```python
from build123d import *

# Parameters (mm, degrees)
SKETCH1_W                                        = 101.6
SKETCH1_H                                        = 50.8
BOSS_EXTRUDE1_DEPTH                              = 25.4
SKETCH2_R                                        = 22.225
CUT_EXTRUDE1_DEPTH                               = 6.35
SKETCH3_R                                        = 9.525
CUT_EXTRUDE2_DEPTH                               = 7.9375
F_1_2_20_TAPPED_HOLE1_D                          = 11.50874
CBORE_FOR_1_2_SOCKET_HEAD_CAP_SCREW1_D           = 13.49248
CBORE_FOR_1_2_SOCKET_HEAD_CAP_SCREW1_CBORE_D     = 20.6375
CBORE_FOR_1_2_SOCKET_HEAD_CAP_SCREW1_CBORE_DEPTH = 12.7


with BuildPart() as part:
    # Sketch1 → Boss-Extrude1 (new body)
    with BuildSketch(Plane(origin=(0, 0, 0), x_dir=(0, 0, -1), z_dir=(1, 0, 0))):
        with Locations((50.8, 25.4)):
            Rectangle(SKETCH1_W, SKETCH1_H)
    extrude(amount=BOSS_EXTRUDE1_DEPTH)

    # Sketch2 → Cut-Extrude1 (cut)
    with BuildSketch(Plane(origin=(0, 50.8, 0), x_dir=(1, 0, 0), z_dir=(0, 1, 0))):
        with Locations((12.7, 50.8)):
            Circle(SKETCH2_R)
    extrude(amount=-CUT_EXTRUDE1_DEPTH, mode=Mode.SUBTRACT)

    # Sketch3 → Cut-Extrude2 (cut)
    with BuildSketch(Plane(origin=(0, 44.45, 0), x_dir=(1, 0, 0), z_dir=(0, 1, 0))):
        with Locations(Location((12.7, 50.8, 0), (0, 0, 270))):
            Circle(SKETCH3_R)
    extrude(amount=-CUT_EXTRUDE2_DEPTH, mode=Mode.SUBTRACT)

    # 1/2-20 Tapped Hole1 (through all)
    with Locations(Plane(origin=(0, 36.5125, 0), x_dir=(1, 0, 0), z_dir=(0, 1, 0))):
        with Locations((12.7, 50.8)):
            Hole(F_1_2_20_TAPPED_HOLE1_D / 2)

    # CBORE for 1/2 Socket Head Cap Screw1 (through all)
    with Locations(Plane(origin=(0, 50.8, 0), x_dir=(1, 0, 0), z_dir=(0, 1, 0))):
        with Locations((12.7, 88.9), (12.7, 12.7)):
            CounterBoreHole(CBORE_FOR_1_2_SOCKET_HEAD_CAP_SCREW1_D / 2, CBORE_FOR_1_2_SOCKET_HEAD_CAP_SCREW1_CBORE_D / 2, CBORE_FOR_1_2_SOCKET_HEAD_CAP_SCREW1_CBORE_DEPTH)


solid = part.part
```
Could you check a few things on this model? Use its own coordinates, in mm. A direction names the side the tool comes from. Coordinates: 2 decimals unless noted, no trailing zeros. Order: outer loops, then holes, each group sorted by start corner. A loop starts at its lowest first (then second) coordinate and runs counter-clockwise, first axis right, second up. Notation, with made-up numbers: M -6,76.25 L 36,76.25 A20 cw 36,92.25 Z; hole C -12,44.25 d4. An arc over 180 degrees is marked long. Use one line per item in the form item = value. Start each with the question number.
1. Suppose I cut it at B-B on z = -88.9. Write out the boundary of the cut face in (x, y).
2. Please list where these lines run through material, in increasing order: line 1 (Z direction, x = 12.7, y = 44.5) (3 decimals); line 2 (Z direction, x = 15.5, y = 6); line 3 (X direction, y = 14.5, z = -88.9).
3. For pin 1 (4 mm diameter, centred on x = 10, z = -47.5, fed in from +Y); pin 2 (4 mm diameter, centred on x = 23, z = -90, fed in from -Y); pin 3 (10.5 mm diameter, centred on x = 12, z = -84.5, fed in from +Y), each with a flat end and sliding along its axis, tell me the tip position at first contact or that it passes through.
4. Suppose I cut it at D-D on y = 16. Write out the boundary of the cut face in (x, z), then the cut area to 3 significant figures.
5. On a 3-axis mill with a long thin cutter (end or side, diameter ignored), from which of +Z, -Z, +X, -X, +Y, -Y can I reach the whole of each face in a straight line? I mean faces 5 (the flat face through (0, 26, -50)), 6 (the cylindrical face through (11.36, 44.54, -99.13)). Say none if no direction works.
6. We'd pull the mould along Z, two halves only. Please class faces 1 (the flat face through (13, 50.8, -78)), 2 (the flat face through (15, 38.1, -82)), 3 (the flat face through (13, 25, 0)), 4 (the cylindrical face through (10.463, 44.539, -2.627)): +Z half, -Z half, draft (parallel to the pull), parting line (faces both ways), or undercut.
7. Suppose I cut it at A-A on y = 47. Count the separate pieces of the cut face and the enclosed holes in it, then the cut area to 3 significant figures.
Geometry says:
q1.outline = M 0,0 L 5.95,0 L 5.95,38.1 L 2.38,38.1 L 2.38,50.8 L 0,50.8 Z; M 19.45,0 L 25.4,0 L 25.4,50.8 L 23.02,50.8 L 23.02,38.1 L 19.45,38.1 Z
q2.line_1 = -101.6 to -99.219, -78.581 to -73.025, -28.575 to -23.019, -2.381 to 0
q2.line_2 = -101.6 to -95.04, -82.76 to -55.83, -45.77 to -18.84, -6.56 to 0
q2.line_3 = 0 to 5.95, 19.45 to 25.4
q3.pin_1 = 36.51
q3.pin_2 = 0
q3.pin_3 = 38.1
q4.outline = M 0,-101.6 L 25.4,-101.6 L 25.4,0 L 0,0 Z; hole C 12.7,-88.9 d13.49; hole C 12.7,-12.7 d13.49; hole C 12.7,-50.8 d11.51
q4.area = 2,190 mm^2
q5.face_5 = +Z, -Z, -X, +Y, -Y
q5.face_6 = +Y
q6.face_1 = draft
q6.face_2 = undercut
q6.face_3 = +Z half
q6.face_4 = undercut
q7.separate_pieces = 2
q7.enclosed_holes = 2
q7.area = 847 mm^2
